from build123d import *

# Parameters (mm, degrees)
SKETCH1_R           = 8
SKETCH1_R_2         = 4
BOSS_EXTRUDE1_DEPTH = 32
SKETCH2_R           = 12.654046274
BOSS_EXTRUDE2_DEPTH = 5
SKETCH3_R           = 15
SKETCH3_R_2         = 10
BOSS_EXTRUDE3_DEPTH = 40
FILLET1_R           = 2.2
SKETCH4_R           = 1.5
CUT_EXTRUDE1_DEPTH  = 20
RIB5_REACH          = 81.869
SKETCH5_WALL_W      = 180.122060892
SKETCH5_WALL_H      = 2
CIRPATTERN1_COUNT   = 4


with BuildPart() as part:
    # Sketch1 → Boss-Extrude1 (new body)
    with BuildSketch(Plane(origin=(0, 0, 0), x_dir=(1, 0, 0), z_dir=(0, 1, 0))):
        with Locations(Location((0, 0, 0), (0, 0, 270))):
            Circle(SKETCH1_R)
        with Locations(Location((0, 0, 0), (0, 0, 270))):
            Circle(SKETCH1_R_2, mode=Mode.SUBTRACT)
    extrude(amount=BOSS_EXTRUDE1_DEPTH)

    # Sketch2 → Boss-Extrude2 (add)
    with BuildSketch(Plane(origin=(0, 32, 0), x_dir=(1, 0, 0), z_dir=(0, 1, 0))):
        with Locations(Location((0, 0, 0), (0, 0, 270))):
            Circle(SKETCH2_R)
    extrude(amount=BOSS_EXTRUDE2_DEPTH)

    # Sketch3 → Boss-Extrude3 (add)
    with BuildSketch(Plane(origin=(0, 37, 0), x_dir=(1, 0, 0), z_dir=(0, 1, 0))):
        with Locations(Location((0, 0, 0), (0, 0, 270))):
            Circle(SKETCH3_R)
        with Locations(Location((0, 0, 0), (0, 0, 270))):
            Circle(SKETCH3_R_2, mode=Mode.SUBTRACT)
    extrude(amount=BOSS_EXTRUDE3_DEPTH)

    # Fillet1
    fillet1_edges = [part.edges().sort_by_distance(p)[0] for p in [
        (0, 37, -12.654046274),
        (0, 32, -8),
        (0, 32, -12.654046274),
    ]]
    fillet(fillet1_edges, radius=FILLET1_R)

    # Sketch4 → Cut-Extrude1 (cut, symmetric)
    with BuildSketch(Plane.XY):
        with Locations((0, 57)):
            Circle(SKETCH4_R)
        with Locations((0, 12)):
            Circle(SKETCH4_R)
    extrude(amount=CUT_EXTRUDE1_DEPTH, both=True, mode=Mode.SUBTRACT)

    # Sketch5 wall → Rib5 (add, up to next)
    with BuildSketch(Plane(origin=(10.5, 28.5, 0), x_dir=(-0.380749805254, -0.924678098475, 0), z_dir=(0.924678098475, -0.380749805254, 0)), mode=Mode.PRIVATE) as rib5_sk1:
        Rectangle(SKETCH5_WALL_W, SKETCH5_WALL_H)
    rib5_tool1 = extrude(rib5_sk1.sketch, amount=-RIB5_REACH, mode=Mode.PRIVATE) - part.part
    rib5 = rib5_tool1.solids().sort_by_distance((10.5, 28.5, 0))[0]
    add(rib5)

    # CirPattern1: Rib5 ×4 about axis
    cirpattern1_axis = Axis((0, 0, 0), (0, 1, 0))
    for i in range(1, CIRPATTERN1_COUNT):
        add(rib5.rotate(cirpattern1_axis, i * 360 / CIRPATTERN1_COUNT))


solid = part.part
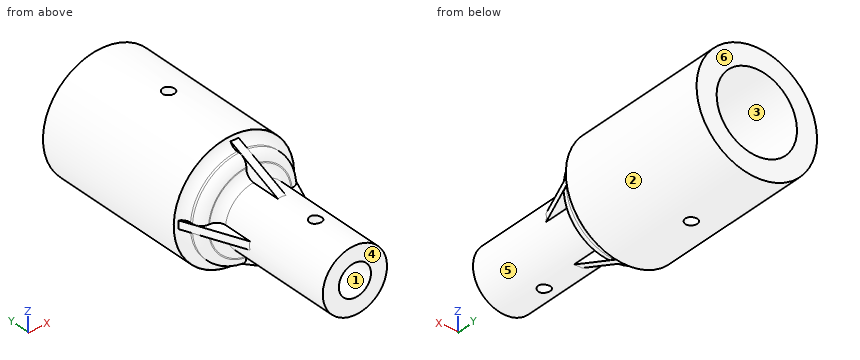
Part model, mm, in its own coordinate system. Face numbers are marked on the shaded views. A direction names the side the tool comes from. Round coordinates to 2 decimals unless told otherwise and drop trailing zeros. Order: outer loops, then holes, each group sorted by start corner. A loop starts at its lowest first (then second) coordinate and runs counter-clockwise, first axis right, second up. Notation, with made-up numbers: (22, 4.25) -> (40, 4.25) arc R26 ccw to (40, 32.25) -> close; hole circle Ø7 at (-5.5, 10.25). An arc over 180 degrees is marked (long way). Put each result on its own line as item: value.
Q1. Band-saw the part on B-B (z = 0). Give the cut face in (x, y).
From the geometry:
outline: (-15, 37) -> (-14.85, 37) arc R2.2 cw to (-13.91, 36.79) -> (-8, 22.43) -> (-8, 0) -> (-4, 0) -> (-4, 32) -> (4, 32) -> (4, 0) -> (8, 0) -> (8, 22.43) -> (13.91, 36.79) arc R2.2 cw to (14.85, 37) -> (15, 37) -> (15, 77) -> (10, 77) -> (10, 37) -> (-10, 37) -> (-10, 77) -> (-15, 77) -> close
Q2. Band-saw the part on C-C (y = 12). Give the cut face in (x, z), and give its area (3 significant figures).
From the geometry:
outline: (-1.5, -7.86) -> (-1.5, -3.71) arc R4 cw to (-1.5, 3.71) -> (-1.5, 7.86) arc R8 ccw to start; (1.5, -7.86) arc R8 ccw to (1.5, 7.86) -> (1.5, 3.71) arc R4 cw to (1.5, -3.71) -> close
area: 127 mm2
Q3. Pin check, flat tips, straight feed: pin 1 Ø6.5 at (y, z) = (28.5, 10) entering from -X; pin 2 Ø6 at (x, z) = (-2.5, -3) entering from +Y; pin 3 Ø3 at (x, y) = (-11, 33) entering from -Z; pin 4 Ø6 at (x, z) = (7.5, 3) entering from -Y. Stop position of each tip, or through.
From the geometry:
pin 1: stops at x = -4.29
pin 2: stops at y = 37
pin 3: stops at z = -8.09
pin 4: stops at y = 0
Q4. Band-saw the part on D-D (x = 0). State how many separate pieces and enclosed holes the cut face has, and give its area (3 significant figures).
From the geometry:
separate pieces: 5
enclosed holes: 0
area: 770 mm2
Q5. Tool access for the marked faces 5 and 6: list every direction of +Z, -Z, +X, -X, +Y, -Y with a clear straight run to the whole face (end or side of a thin tool).
From the geometry:
face 5: -Y
face 6: +Z, -Z, +X, -X, +Y
Q6. Wall check: line 1 (X direction, y = 59, z = 0); line 2 (Z direction, x = 0, y = 17). Give the ranges that are in metal, low to high. Write a range as [from, to].
From the geometry:
line 1: x = [-15, -10], [10, 15]
line 2: z = [-8, -4], [4, 8]
Q7. Pull direction Z, two halves, no side cores. Call the marked faces 1, 2, 3 and 4: pulls with the +Z half, pulls with the -Z half, needs draft (parallel to the pull), parting line crosses it, or undercut.
From the geometry:
face 1: undercut
face 2: parting line crosses it
face 3: undercut
face 4: needs draft
